```python
from build123d import *

# Parameters (mm, degrees)
SKETCH1_W           = 88.9
SKETCH1_H           = 88.9
BOSS_EXTRUDE1_DEPTH = 6.35
SKETCH2_R           = 9.525
SKETCH2_W           = 18.288
SKETCH2_H           = 5.588
SKETCH2_W_2         = 5.588
SKETCH2_H_2         = 18.288
CUT_EXTRUDE1_DEPTH  = 126.88384527
SKETCH3_W           = 19.05
SKETCH3_H           = 6.35
SKETCH3_W_2         = 6.35
SKETCH3_H_2         = 19.05
CUT_EXTRUDE2_DEPTH  = 126.88384527
CUT_EXTRUDE3_DEPTH  = 126.88384527


with BuildPart() as part:
    # Sketch1 → Boss-Extrude1 (new body)
    with BuildSketch(Plane(origin=(0, 0, 0), x_dir=(1, 0, 0), z_dir=(0, 1, 0))):
        with Locations((44.45, 44.45)):
            Rectangle(SKETCH1_W, SKETCH1_H)
    extrude(amount=BOSS_EXTRUDE1_DEPTH)

    # Sketch2 → Cut-Extrude1 (cut, through all)
    with BuildSketch(Plane(origin=(0, 6.35, 0), x_dir=(1, 0, 0), z_dir=(0, 1, 0))):
        with Locations(Location((44.45, 44.45, 0), (0, 0, 270))):
            Circle(SKETCH2_R)
        with Locations((44.45, 73.406)):
            Rectangle(SKETCH2_W, SKETCH2_H)
        with Locations((16.256, 44.45)):
            Rectangle(SKETCH2_W_2, SKETCH2_H_2)
        with Locations((72.644, 44.45)):
            Rectangle(SKETCH2_W_2, SKETCH2_H_2)
        with Locations((44.45, 15.494)):
            Rectangle(SKETCH2_W, SKETCH2_H)
    extrude(amount=-CUT_EXTRUDE1_DEPTH, mode=Mode.SUBTRACT)

    # Sketch3 → Cut-Extrude2 (cut, through all)
    with BuildSketch(Plane(origin=(0, 6.35, 0), x_dir=(1, 0, 0), z_dir=(0, 1, 0))):
        with Locations((44.45, 85.725)):
            Rectangle(SKETCH3_W, SKETCH3_H)
        with Locations((85.725, 44.45)):
            Rectangle(SKETCH3_W_2, SKETCH3_H_2)
        with Locations((44.45, 3.175)):
            Rectangle(SKETCH3_W, SKETCH3_H)
        with Locations((3.175, 44.45)):
            Rectangle(SKETCH3_W_2, SKETCH3_H_2)
    extrude(amount=-CUT_EXTRUDE2_DEPTH, mode=Mode.SUBTRACT)

    # Sketch4 → Cut-Extrude3 (cut, through all)
    with BuildSketch(Plane(origin=(0, 6.35, 0), x_dir=(1, 0, 0), z_dir=(0, 1, 0))):
        Polygon((23.495, 46.0375), (23.495, 48.26), (26.67, 48.26), (26.67, 46.249166667), (27.432, 46.249166667), (27.432, 42.650833333), (26.67, 42.650833333), (26.67, 40.64), (23.495, 40.64), (23.495, 42.8625), (6.35, 42.8625), (6.35, 46.0375), align=None)
        Polygon((62.23, 46.249166667), (61.468, 46.249166667), (61.468, 42.650833333), (62.23, 42.650833333), (62.23, 40.64), (65.405, 40.64), (65.405, 42.8625), (82.55, 42.8625), (82.55, 46.0375), (65.405, 46.0375), (65.405, 48.26), (62.23, 48.26), align=None)
    extrude(amount=-CUT_EXTRUDE3_DEPTH, mode=Mode.SUBTRACT)


solid = part.part
```
Build history of the part. All positions in model axes, mm. A direction names the side the tool comes from. Give positions to 0.01 mm unless a question says otherwise; leave off trailing zeros. Loops run counter-clockwise (first coordinate to the right, second up) from the corner with the lowest first, then second, coordinate; pieces in that order, holes last. Notation, with made-up numbers: (73.5, 85) - (101.5, 85) arc R11 ccw to (101.5, 90) - close; hole circle Ø9 at (50.25, -30.75). An arc over 180 degrees is marked (long way). Use a Markdown table: item, result.
(1) Which spindle directions (+Z, -Z, +X, -X, +Y, -Y) get a long thin tool onto all of the face, cutting with end or side? Do faces 5 (the face through (13.462, 3, -50)), 6 (the face through (68, 3, -46.038)), 7 (the face through (53.975, 3, -3)), 8 (the face through (10, 3, -46.038)). Say none if no direction does.
Taken from the geometry:
| item | result |
|---|---|
| face 5 | +Y, -Y |
| face 6 | +X, +Y, -Y |
| face 7 | +Z, +Y, -Y |
| face 8 | -X, +Y, -Y |
(2) Wall check: line 1 along X through (y, z) = (2, -14); line 2 along Z through (x, y) = (19, 2.25); line 3 along Z through (x, y) = (69, 5.5). Give the ranges that are in metal, low to high.
Taken from the geometry:
| item | result |
|---|---|
| line 1 | 0 to 35.31, 53.59 to 88.9 |
| line 2 | -88.9 to -53.59, -35.31 to 0 |
| line 3 | -88.9 to -46.04, -42.86 to 0 |
(3) Band-saw the part on B-B (z = -75). Give the cut face in (x, y).
Taken from the geometry:
| item | result |
|---|---|
| outline | (0, 0) - (35.31, 0) - (35.31, 6.35) - (0, 6.35) - close; (53.59, 0) - (88.9, 0) - (88.9, 6.35) - (53.59, 6.35) - close |
(4) Band-saw the part on D-D (y = 4.75). Give the number of separate pieces and of enclosed holes in the cut face, and give its area (3 significant figures).
Taken from the geometry:
| item | result |
|---|---|
| separate pieces | 1 |
| enclosed holes | 3 |
| area | 6,600 mm2 |
(5) Drop flat-ended pins along their axis: pin 1 Ø1.1 at (y, z) = (3.5, -41.5) entering from +X; pin 2 Ø11.5 at (x, z) = (44.45, -44.45) entering from +Y. Give the stop position or say it passes through.
Taken from the geometry:
| item | result |
|---|---|
| pin 1 | x = 82.55 |
| pin 2 | through |
(6) Band-saw the part on C-C (x = 44.45). Give the cut face in (y, z) (3 decimals), and give its area (3 significant figures).
Taken from the geometry:
| item | result |
|---|---|
| outline | (0, -82.55) - (6.35, -82.55) - (6.35, -76.2) - (0, -76.2) - close; (0, -70.612) - (6.35, -70.612) - (6.35, -53.975) - (0, -53.975) - close; (0, -34.925) - (6.35, -34.925) - (6.35, -18.288) - (0, -18.288) - close; (0, -12.7) - (6.35, -12.7) - (6.35, -6.35) - (0, -6.35) - close |
| area | 292 mm2 |
(7) Band-saw the part on A-A (x = 81.5). Give the cut face in (y, z), and give its area (3 significant figures).
Taken from the geometry:
| item | result |
|---|---|
| outline | (0, -88.9) - (6.35, -88.9) - (6.35, -46.04) - (0, -46.04) - close; (0, -42.86) - (6.35, -42.86) - (6.35, 0) - (0, 0) - close |
| area | 544 mm2 |
(8) Pull direction X, two halves, no side cores. Call faces 1 (the face through (0, 3, -17)), 2 (the face through (88.9, 3, -71)), 3 (the face through (3, 3, -53.975)), 4 (the face through (34.925, 3, -86)): +X half, -X half, draft (parallel to the pull), parting line (faces both ways), or undercut.
Taken from the geometry:
| item | result |
|---|---|
| face 1 | -X half |
| face 2 | +X half |
| face 3 | draft |
| face 4 | undercut |
